Read the model definition and answer for the solid it produces. Units are mm, in the model's axes. A direction names the side the tool comes from. Give positions to 0.01 mm unless a question says otherwise; leave off trailing zeros. Loops run counter-clockwise (first coordinate to the right, second up) from the corner with the lowest first, then second, coordinate; pieces in that order, holes last. Notation, with made-up numbers: (34, 15) - (80, 15) arc R15 cw to (80, 34) - close; hole circle Ø3 at (26, -0.5). An arc over 180 degrees is marked (long way). Write item = value, one per line.
```python
from build123d import *

# Parameters (mm, degrees)
SKETCH_1_W          = 102
SKETCH_1_H          = 70
EXTRUDE_1_DEPTH     = 5
SKETCH_2_R          = 1
CUT_EXTRUDE_1_DEPTH = 4.5
SKETCH_3_W          = 7
SKETCH_3_H          = 1
CUT_EXTRUDE_2_DEPTH = 2
SKETCH_4_W          = 80
SKETCH_4_H          = 35
CUT_EXTRUDE_3_DEPTH = 5
SKETCH_5_W          = 11
SKETCH_5_H          = 35
CUT_EXTRUDE_4_DEPTH = 1
SKETCH_6_W          = 100
SKETCH_6_H          = 68
CUT_EXTRUDE_5_DEPTH = 1


with BuildPart() as part:
    # Эскиз1 → Бобышка-Вытянуть1 (new body)
    with BuildSketch(Plane(origin=(0, 0, 0), x_dir=(1, 0, 0), z_dir=(0, 1, 0))):
        Rectangle(SKETCH_1_W, SKETCH_1_H)
    extrude(amount=EXTRUDE_1_DEPTH)

    # Эскиз2 → Вырез-Вытянуть1 (cut)
    with BuildSketch(Plane(origin=(0, 5, 0), x_dir=(1, 0, 0), z_dir=(0, 1, 0))):
        with Locations(Location((-46, 31.5, 0), (0, 0, 270))):
            Circle(SKETCH_2_R)
        with Locations(Location((33, 31.5, 0), (0, 0, 90))):
            Circle(SKETCH_2_R)
        with Locations(Location((33, -31.5, 0), (0, 0, 270))):
            Circle(SKETCH_2_R)
        with Locations(Location((-46, -31.5, 0), (0, 0, 90))):
            Circle(SKETCH_2_R)
    extrude(amount=-CUT_EXTRUDE_1_DEPTH, mode=Mode.SUBTRACT)

    # Эскиз3 → Вырез-Вытянуть2 (cut)
    with BuildSketch(Plane.ZY.offset(51)):
        with Locations((0, 4.5)):
            Rectangle(SKETCH_3_W, SKETCH_3_H)
    extrude(amount=-CUT_EXTRUDE_2_DEPTH, mode=Mode.SUBTRACT)

    # Эскиз4 → Вырез-Вытянуть3 (cut)
    with BuildSketch(Plane.XZ):
        Rectangle(SKETCH_4_W, SKETCH_4_H)
    extrude(amount=-CUT_EXTRUDE_3_DEPTH, mode=Mode.SUBTRACT)

    # Эскиз5 → Вырез-Вытянуть4 (cut)
    with BuildSketch(Plane.XZ):
        with Locations((45.5, 0)):
            Rectangle(SKETCH_5_W, SKETCH_5_H)
    extrude(amount=-CUT_EXTRUDE_4_DEPTH, mode=Mode.SUBTRACT)

    # Эскиз6 → Вырез-Вытянуть5 (cut)
    with BuildSketch(Plane(origin=(0, 5, 0), x_dir=(1, 0, 0), z_dir=(0, 1, 0))):
        Rectangle(SKETCH_6_W, SKETCH_6_H)
    extrude(amount=-CUT_EXTRUDE_5_DEPTH, mode=Mode.SUBTRACT)


solid = part.part
```
1) A tool of negligible diameter and unlimited length cuts with its end or side. For faces 1 (the face through (45, 1, 0)), 2 (the face through (40, 2, 0)), 3 (the face through (33.99, 2.27, 31.37)), from which of +Z, -Z, +X, -X, +Y, -Y can it reach the whole face along a straight path? Write none if from no direction.
Output:
face_1 = +X, -Y
face_2 = +Y, -Y
face_3 = +Y
2) A cutting plane is placed at B-B on x = 33. Determine the outline of the cut face in (y, z), then the cut area to 3 significant figures.
Output:
outline = (0, -35) - (5, -35) - (5, -34) - (4, -34) - (4, -32.5) - (0.5, -32.5) - (0.5, -30.5) - (4, -30.5) - (4, -17.5) - (0, -17.5) - close; (0, 17.5) - (4, 17.5) - (4, 30.5) - (0.5, 30.5) - (0.5, 32.5) - (4, 32.5) - (4, 34) - (5, 34) - (5, 35) - (0, 35) - close
area = 128 mm²
3) A cutting plane is placed at A-A on z = -9.5. Determine the outline of the cut face in (x, y).
Output:
outline = (-51, 0) - (-40, 0) - (-40, 4) - (-50, 4) - (-50, 5) - (-51, 5) - close; (40, 1) - (51, 1) - (51, 5) - (50, 5) - (50, 4) - (40, 4) - close
4) A cutting plane is placed at C-C on x = -46. Determine the outline of the cut face in (y, z), then the cut area to 3 significant figures.
Output:
outline = (0, -35) - (5, -35) - (5, -34) - (4, -34) - (4, -32.5) - (0.5, -32.5) - (0.5, -30.5) - (4, -30.5) - (4, 30.5) - (0.5, 30.5) - (0.5, 32.5) - (4, 32.5) - (4, 34) - (5, 34) - (5, 35) - (0, 35) - close
area = 268 mm²
5) A cutting plane is placed at D-D on x = 4. Determine the outline of the cut face in (y, z).
Output:
outline = (0, -35) - (5, -35) - (5, -34) - (4, -34) - (4, -17.5) - (0, -17.5) - close; (0, 17.5) - (4, 17.5) - (4, 34) - (5, 34) - (5, 35) - (0, 35) - close
6) Find the intervals of material crossed by probe 1 along X at (y, z) = (2, -31.5); probe 2 along X at (y, z) = (2.2, 6); probe 3 along Y at (x, z) = (-43.5, 30), in increasing order.
Output:
probe_1 = -51 to -47, -45 to 32, 34 to 51
probe_2 = -51 to -40, 40 to 51
probe_3 = 0 to 4
7) Each of these flat-tipped pins is pushed along its axis until it touches: P1, Ø1.6, axis at x = -46.5, z = 31.5, coming from the +Y side; P2, Ø1.2, axis at x = 33, z = 31.5, coming from the +Y side; P3, Ø8, axis at x = -28, z = -14.5, coming from the -Y side. Where does it stop, or does it pass through?
Output:
P1 = 4
P2 = 0.5
P3 = 0
8) The mould has two halves that part along Z. Classify faces 4 (the face through (51, 2, 0)), 5 (the face through (-1, 2, 35)), 6 (the face through (32.01, 2.27, -31.37)): pulls with the +Z half, pulls with the -Z half, needs draft (parallel to the pull), parting line crosses it, or undercut.
Output:
face_4 = needs draft
face_5 = pulls with the +Z half
face_6 = undercut
